For this review, take the finished solid that the model builds, in its own axes (mm). Face numbers are marked on the shaded views. A direction names the side the tool comes from. Coordinates: 2 decimals unless noted, no trailing zeros. Write each loop counter-clockwise with the first axis right and the second up, starting at its lowest first coordinate (ties: lowest second). Pieces come first, ordered by that corner, then holes.
1) For the marked faces 1 and 2, list the 3-axis set-ups (+Z, -Z, +X, -X, +Y, -Y) from which the entire face can be reached by the end or side of a thin tool; tool diameter is ignored.
2) Insertion check: P1, Ø12, axis at x = -20, z = 4.5, coming from the +Y side; P2, Ø1.2, axis at x = -17, y = 10, coming from the -Z side; P3, Ø3.5, axis at x = -24, z = -27, coming from the +Y side. Each pin has a flat end and moves straight along its axis. Give the tip position at first contact, or say it passes through.
3) We need section C-C on x = 5. Write out the cut boundary in (y, z).
4) We need section D-D on z = 9. Write out the cut boundary in (x, y).
5) Mouldability with a two-part tool opening along X and no side actions: class the marked faces 3, 4 and 5 as pulls with the +X half, pulls with the -X half, needs draft (parallel to the pull), parting line crosses it, or undercut.
6) To check wall thickness, follow line 1 along X through (y, z) = (0.8, -27.5); line 2 along Z through (x, y) = (46.5, 1.3); line 3 along Y through (x, z) = (-37.5, -8). State the ranges of each line that lie inside material, in increasing order.
7) We need section B-B on z = -27.5. Give the number of separate pieces and of enclosed holes in the cut face, then the cut area to 3 significant figures.
8) We need section A-A on x = -46.5. Write out the cut boundary in (y, z).
Autodesk Inventor part; units mm, degrees
ref_plane "Work Plane1" through (-49, 0, 0) normal (1, 0, 0) x (0, 1, 0)
ref_plane "XZ Plane" through (0, 0, 0) normal (0, 1, 0) x (-1, 0, 0)
ref_plane "XY Plane" through (0, 0, 0) normal (0, 0, 1) x (1, 0, 0)
ref_plane "Work Plane1" through (-49, 0, 0) normal (1, 0, 0) x (0, 1, 0)
sketch "Sketch1" plane through (-49, 0, 0) normal (1, 0, 0) x (0, 1, 0)
  line L0 (1.5875, -30) -> (1.5875, 30)
  line L1 (1.5875, 30) -> (0, 30)
  line L2 (0, -30) -> (0, 30)
  line L3 (1.5875, -30) -> (0, -30)
  dimension "d44" = 1.5875
  dimension "d45" = 60
extrude "Extrusion3" add sketch "Sketch1" along normal blind 98 draft 0
sketch "Sketch3" plane through (-49, 1.5875, 30) normal (0, 1, 0) x (1, 0, 0)
  line L0 (97.5, 50) -> (0.5, 50)
  line L1 (0.5, 50) -> (0.5, 10.5)
  line L2 (97.5, 10.5) -> (97.5, 50)
  line L3 (0.5, 10.5) -> (97.5, 10.5)
extrude "Extrusion2" add sketch "Sketch3" along normal blind 9
sketch "Sketch4" plane through (-49, 10.5875, 30) normal (0, 1, 0) x (1, 0, 0)
  line L0 (87, 17.25) -> (87, 43.25)
  line L1 (11, 17.25) -> (87, 17.25)
  line L2 (11, 43.25) -> (11, 17.25)
  line L3 (87, 43.25) -> (11, 43.25)
extrude "Extrusion1" cut sketch "Sketch4" against normal blind 1.5
hole "Hole4" at (-46.5, 1.5875, 27.5) direction (0, -1, 0) diameter 3 depth 1.5875
hole "Hole3" at (46.5, 1.5875, 27.5) direction (0, -1, 0) diameter 3 depth 1.5875
sketch "Sketch6" plane through (-49, 1.5875, 30) normal (0, 1, 0) x (1, 0, 0)
  point P0 (95.5, 2.5)
hole "Hole2" at (46.5, 1.5875, -27.5) direction (0, -1, 0) diameter 3 depth 1.5875
sketch "Sketch5" plane through (-49, 1.5875, 30) normal (0, 1, 0) x (1, 0, 0)
  point P0 (2.5, 2.5)
hole "Hole1" at (-46.5, 1.5875, -27.5) direction (0, -1, 0) diameter 3 depth 1.5875
fillet "Fillet4" radius 2 1 edges at (-38, 9.8375, -13.25)
fillet "Fillet3" radius 2 1 edges at (-38, 9.8375, 12.75)
fillet "Fillet2" radius 2 1 edges at (38, 9.8375, 12.75)
fillet "Fillet1" radius 2 1 edges at (38, 9.8375, -13.25)
sketch "Sketch9" plane through (-49, 1.5875, 30) normal (0, 1, 0) x (1, 0, 0)
  line L0 (0, 60) -> (98, 60)
  line L1 (9.045, 60) -> (46.854, 60)
  line L2 (46.854, 60) -> (46.854, 55.474)
  line L3 (46.854, 55.474) -> (9.045, 55.474)
  line L4 (9.045, 55.474) -> (9.045, 60)
  line L5 (0, 60) -> (0, 0)
  point P0 (49, 30)
  dimension "d41" = 37.809
  dimension "d42" = 4.526
  dimension "d43" = 9.045
extrude "Extrusion4" add sketch "Sketch9" along normal blind 0.0356
sketch "Sketch7" plane through (-49, 1.5875, 30) normal (0, 1, 0) x (1, 0, 0)
  point P0 (95.5, 57.5)
sketch "Sketch8" plane through (-49, 1.5875, 30) normal (0, 1, 0) x (1, 0, 0)
  point P0 (2.5, 57.5)
properties part number "4x20 LCD"
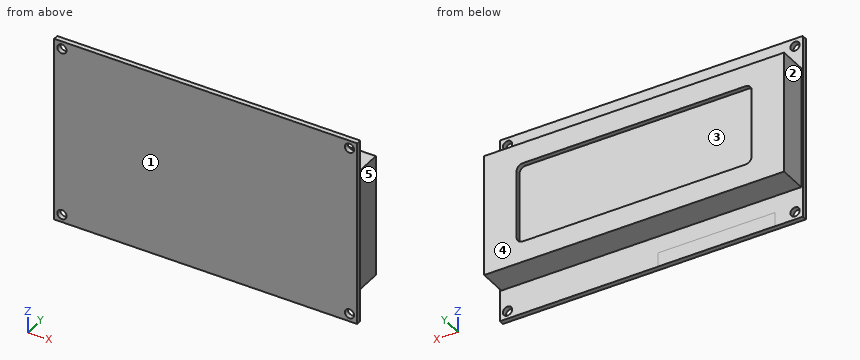
Result:
1. face 1: +Z, -Z, +X, -X, -Y
1. face 2: +Z, -Z, -X, +Y
2. P1: stops at y = 9.09
2. P2: stops at z = -20
2. P3: stops at y = 1.62
3. outline: (0, -30) - (1.59, -30) - (1.59, -20) - (10.59, -20) - (10.59, -13.25) - (9.09, -13.25) - (9.09, 12.75) - (10.59, 12.75) - (10.59, 19.5) - (1.59, 19.5) - (1.59, 30) - (0, 30) - close
4. outline: (-49, 0) - (49, 0) - (49, 1.59) - (48.5, 1.59) - (48.5, 10.59) - (38, 10.59) - (38, 9.09) - (-38, 9.09) - (-38, 10.59) - (-48.5, 10.59) - (-48.5, 1.59) - (-49, 1.59) - close
5. face 3: undercut
5. face 4: needs draft
5. face 5: pulls with the +X half
6. line 1: x = -49 to -48, -45 to 45, 48 to 49
6. line 2: z = -30 to -29, -26 to 26, 29 to 30
6. line 3: y = 0 to 9.09
7. separate pieces: 3
7. enclosed holes: 0
7. area: 147 mm2
8. outline: (0, -30) - (1.59, -30) - (1.59, -29) - (0, -29) - close; (0, -26) - (1.59, -26) - (1.59, -20) - (10.59, -20) - (10.59, 19.5) - (1.59, 19.5) - (1.59, 26) - (0, 26) - close; (0, 29) - (1.59, 29) - (1.59, 30) - (0, 30) - close
